from build123d import *

# Parameters (mm, degrees)
EXTRUDE_1_DEPTH                = 40
FILLET_1_R                     = 0.25
FILLET_2_R                     = 0.5
SKETCH_2_R                     = 1.5
CUT_EXTRUDE_1_DEPTH            = 2.3
SKETCH_3_R                     = 1.2
CUT_EXTRUDE_2_DEPTH            = 41.684763733
FILLET_3_R                     = 0.5
PATTERN_LINEAR_2_COUNT         = 3
PATTERN_LINEAR_2_PITCH         = 15
FILLET_3_OF_PATTERN_LINEAR_2_R = 0.5


with BuildPart() as part:
    # 草图1 → 凸台-拉伸1 (new body)
    with BuildSketch(Plane.XY):
        Polygon((7, 2.5), (7, 0), (0, 0), (0, 2.5), (1, 2.5), (1, 3.5), (0, 3.5), (0, 4.8), (7, 4.8), (7, 3.5), (6, 3.5), (6, 2.5), align=None)
    extrude(amount=EXTRUDE_1_DEPTH)

    # 圆角1
    fillet_1_edges = [part.edges().sort_by_distance(p)[0] for p in [
        (0, 2.5, 20),
        (1, 2.5, 20),
        (1, 3.5, 20),
        (0, 3.5, 20),
        (0, 4.8, 20),
        (7, 4.8, 20),
        (7, 3.5, 20),
        (6, 3.5, 20),
        (6, 2.5, 20),
        (7, 2.5, 20),
    ]]
    fillet(fillet_1_edges, radius=FILLET_1_R)

    # 圆角2
    fillet_2_edges = [part.edges().sort_by_distance(p)[0] for p in [
        (7, 0, 20),
        (0, 0, 20),
    ]]
    fillet(fillet_2_edges, radius=FILLET_2_R)

    # 草图2 → 切除-拉伸1 (cut)
    with BuildSketch(Plane(origin=(0, 4.8, 0), x_dir=(1, 0, 0), z_dir=(0, 1, 0))):
        with Locations(Location((3.5, -5, 0), (0, 0, 270))):
            Circle(SKETCH_2_R)
    cut_extrude_1 = extrude(amount=-CUT_EXTRUDE_1_DEPTH, mode=Mode.SUBTRACT)

    # 草图3 → 切除-拉伸2 (cut, through all)
    with BuildSketch(Plane(origin=(0, 2.5, 0), x_dir=(1, 0, 0), z_dir=(0, 1, 0))):
        with Locations(Location((3.5, -5, 0), (0, 0, 270))):
            Circle(SKETCH_3_R)
    cut_extrude_2 = extrude(amount=-CUT_EXTRUDE_2_DEPTH, mode=Mode.SUBTRACT)

    # 圆角3
    fillet_3_edges = [part.edges().sort_by_distance(p)[0] for p in [
        (3.5, 4.8, 3.5),
    ]]
    fillet(fillet_3_edges, radius=FILLET_3_R)

    # 阵列(线性)2: 切除-拉伸1, 切除-拉伸2 ×3
    with Locations(*[(0, 0, i * PATTERN_LINEAR_2_PITCH) for i in range(1, PATTERN_LINEAR_2_COUNT)]):
        add(cut_extrude_1, mode=Mode.SUBTRACT)
        add(cut_extrude_2, mode=Mode.SUBTRACT)

    # 圆角3 of 阵列(线性)2
    fillet_3_of_pattern_linear_2_edges = [part.edges().sort_by_distance(p)[0] for p in [
        (3.5, 4.8, 18.5),
        (3.5, 4.8, 33.5),
    ]]
    fillet(fillet_3_of_pattern_linear_2_edges, radius=FILLET_3_OF_PATTERN_LINEAR_2_R)


solid = part.part
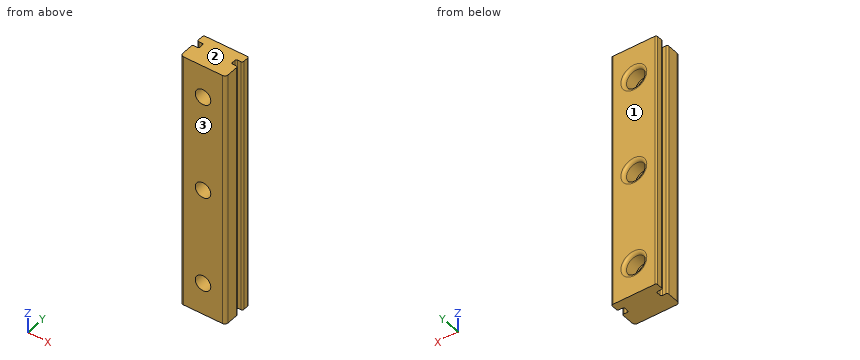
Check sheet for the modelled part. Datum: model origin and axes. Units: mm. Face numbers are marked on the shaded views. Give positions to 0.01 mm unless a question says otherwise; leave off trailing zeros. Order: outer loops, then holes, each group sorted by start corner. A loop starts at its lowest first (then second) coordinate and runs counter-clockwise, first axis right, second up. Notation, with made-up numbers: (-10.5, 18) - (25.5, 18) arc R31 cw to (25.5, 47) - close; hole circle Ø4 at (-25, -40). An arc over 180 degrees is marked (long way). Answer as CSV lines item,"result".
1. Section check D-D (z = 29.5). Record the boundary of the cut face in (x, y), then the cut area to 3 significant figures.
Result sheet:
outline,"(0, 0.5) arc R0.5 ccw to (0.5, 0) - (6.5, 0) arc R0.5 ccw to (7, 0.5) - (7, 2.25) arc R0.25 ccw to (6.75, 2.5) - (6.25, 2.5) arc R0.25 cw to (6, 2.75) - (6, 3.25) arc R0.25 cw to (6.25, 3.5) - (6.75, 3.5) arc R0.25 ccw to (7, 3.75) - (7, 4.55) arc R0.25 ccw to (6.75, 4.8) - (0.25, 4.8) arc R0.25 ccw to (0, 4.55) - (0, 3.75) arc R0.25 ccw to (0.25, 3.5) - (0.75, 3.5) arc R0.25 cw to (1, 3.25) - (1, 2.75) arc R0.25 cw to (0.75, 2.5) - (0.25, 2.5) arc R0.25 ccw to (0, 2.25) - close"
area,"31.5 mm²"
2. Section check B-B (x = 3.5). State how many separate pieces and enclosed holes the cut face has, then the cut area to 3 significant figures.
Result sheet:
separate pieces,"4"
enclosed holes,"0"
area,"153 mm²"
3. Go/stop test with a flat-tipped pin: P1, Ø1.5, axis at x = 3, z = 20, coming from the +Y side. Record where the tip stops, or that it passes through.
Result sheet:
P1,"y = 2.5"
4. Scan lines: probe 1 along X at (y, z) = (3.8, 20); probe 2 along X at (y, z) = (3.15, 35); probe 3 along Z at (x, y) = (4.5, 2.9). Record each from-to range of solid material in increasing order. Write a range as from..to.
Result sheet:
probe 1,"0..2, 5..7"
probe 2,"1..2, 5..6"
probe 3,"0..3.88, 6.12..18.88, 21.12..33.88, 36.12..40"
5. Section check C-C (y = 1.75). Record the boundary of the cut face in (x, z).
Result sheet:
outline,"(0, 0) - (7, 0) - (7, 40) - (0, 40) - close; hole circle Ø2.4 at (3.5, 5); hole circle Ø2.4 at (3.5, 20); hole circle Ø2.4 at (3.5, 35)"
6. Mould release check, pull along Y, two halves, no side actions. Record for the marked faces 1, 2 and 3: released by +Y, released by -Y, zero draft, split by the parting line, or undercut.
Result sheet:
face 1,"released by +Y"
face 2,"zero draft"
face 3,"released by -Y"
